The listing builds one solid part. Answer for the finished solid, in the listing's coordinates (mm). Give positions to 0.01 mm unless a question says otherwise; leave off trailing zeros. Write each loop counter-clockwise with the first axis right and the second up, starting at its lowest first coordinate (ties: lowest second). Pieces come first, ordered by that corner, then holes. Notation, with made-up numbers: (15, -36.75) - (51, -36.75) arc R20 ccw to (51, -8.75) - close; hole circle Ø5 at (-14.5, 13.25). An arc over 180 degrees is marked (long way). Return JSON: item names as keys, results as strings.
from build123d import *

# Parameters (mm, degrees)
SKETCH1_W           = 46
SKETCH1_H           = 50
BOSS_EXTRUDE1_DEPTH = 2
SKETCH2_R           = 11.5
CUT_EXTRUDE2_DEPTH  = 35.029399054
SKETCH3_R           = 1.5
CUT_EXTRUDE3_DEPTH  = 35.029399054


with BuildPart() as part:
    # Sketch1 → Boss-Extrude1 (new body)
    with BuildSketch(Plane(origin=(0, 0, 0), x_dir=(1, 0, 0), z_dir=(0, 1, 0))):
        Rectangle(SKETCH1_W, SKETCH1_H)
    extrude(amount=BOSS_EXTRUDE1_DEPTH)

    # Sketch2 → Cut-Extrude2 (cut, through all)
    with BuildSketch(Plane(origin=(0, 2, 0), x_dir=(1, 0, 0), z_dir=(0, 1, 0))):
        with Locations(Location((0, 0, 0), (0, 0, 270))):
            Circle(SKETCH2_R)
    extrude(amount=-CUT_EXTRUDE2_DEPTH, mode=Mode.SUBTRACT)

    # Sketch3 → Cut-Extrude3 (cut, through all)
    with BuildSketch(Plane(origin=(0, 2, 0), x_dir=(1, 0, 0), z_dir=(0, 1, 0))):
        with Locations(Location((9.899494937, 9.899494937, 0), (0, 0, 270))):
            Circle(SKETCH3_R)
        with Locations(Location((-9.899494937, 9.899494937, 0), (0, 0, 270))):
            Circle(SKETCH3_R)
        with Locations(Location((-9.899494937, -9.899494937, 0), (0, 0, 270))):
            Circle(SKETCH3_R)
        with Locations(Location((9.899494937, -9.899494937, 0), (0, 0, 270))):
            Circle(SKETCH3_R)
    extrude(amount=-CUT_EXTRUDE3_DEPTH, mode=Mode.SUBTRACT)


solid = part.part
Item 1: Consider L1, parallel to X at y = 0.65, z = 0; L2, parallel to X at y = 0.2, z = -1.5; L3, parallel to Z at x = -10.5, y = 0.8. Determine where each line is inside the solid, lowest interval first.
Answer below:
{"L1": "x = -23 to -11.5, 11.5 to 23", "L2": "x = -23 to -11.4, 11.4 to 23", "L3": "z = -25 to -11.27, -8.52 to -4.69, 4.69 to 8.52, 11.27 to 25"}
Item 2: A cutting plane is placed at C-C on y = 1. Determine the outline of the cut face in (x, z).
Answer below:
{"outline": "(-23, -25) - (23, -25) - (23, 25) - (-23, 25) - close; hole circle Ø23 at (0, 0); hole circle Ø3 at (-9.9, -9.9); hole circle Ø3 at (-9.9, 9.9); hole circle Ø3 at (9.9, -9.9); hole circle Ø3 at (9.9, 9.9)"}
Item 3: A cutting plane is placed at A-A on x = 0. Determine the outline of the cut face in (y, z).
Answer below:
{"outline": "(0, -25) - (2, -25) - (2, -11.5) - (0, -11.5) - close; (0, 11.5) - (2, 11.5) - (2, 25) - (0, 25) - close"}
Item 4: A cutting plane is placed at B-B on z = 0. Determine the outline of the cut face in (x, y), then the cut area to 3 significant figures.
Answer below:
{"outline": "(-23, 0) - (-11.5, 0) - (-11.5, 2) - (-23, 2) - close; (11.5, 0) - (23, 0) - (23, 2) - (11.5, 2) - close", "area": "46.0 mm²"}
Item 5: The mould has two halves that part along Z. Classify faces 1 (the face through (0, 1, -25)), 2 (the face through (0, 1, 25)), 3 (the face through (-11, 2, -6)), 4 (the face through (-8.635, 1.014, -9.093)): +Z half, -Z half, draft (parallel to the pull), parting line (faces both ways), or undercut.
Answer below:
{"face 1": "-Z half", "face 2": "+Z half", "face 3": "draft", "face 4": "undercut"}
